The listing builds one solid part. Answer for the finished solid, in the listing's coordinates (mm). Face numbers are marked on the shaded views. A direction names the side the tool comes from. Coordinates: 2 decimals unless noted, no trailing zeros. Order: outer loops, then holes, each group sorted by start corner. A loop starts at its lowest first (then second) coordinate and runs counter-clockwise, first axis right, second up. Notation, with made-up numbers: (-27, 68.25) -> (27, 68.25) arc R24 ccw to (27, 100.25) -> close; hole circle Ø9 at (-5, 8.25). An arc over 180 degrees is marked (long way). One line per question, with ' | ' between items.
Autodesk Inventor part; units mm, degrees
ref_plane "YZ Plane" through (0, 0, 0) normal (1, 0, 0) x (0, 1, 0)
ref_plane "XZ Plane" through (0, 0, 0) normal (0, 1, 0) x (-1, 0, 0)
ref_plane "XY Plane" through (0, 0, 0) normal (0, 0, 1) x (1, 0, 0)
sketch "Sketch1" plane through (0, 0, 0) normal (0, 1, 0) x (-1, 0, 0)
  line L0 (-6, 6) -> (6, 6)
  line L1 (6, 6) -> (6, -6)
  line L2 (6, -6) -> (-6, -6)
  line L3 (-6, -6) -> (-6, 6)
  line L4 (-6, 6) -> (6, -6) construction
  line L5 (6, 6) -> (-6, -6) construction
  line L6 (6, 6) -> (16, 6)
  line L7 (16, -6) -> (6, -6)
  line L8 (6, -6) -> (6, 6)
  line L9 (0, 6) -> (0, -6) construction
  line L10 (-6, 6) -> (-16, 6)
  line L11 (-16, 6) -> (-16, -6)
  line L12 (-16, -6) -> (-6, -6)
  line L13 (-6, -6) -> (-6, -16)
  line L14 (-6, -16) -> (6, -16)
  line L15 (6, -16) -> (6, -6)
  line L16 (6, 6) -> (6, 16)
  line L17 (6, 16) -> (-6, 16)
  line L18 (-6, 16) -> (-6, 6)
  line L19 (16, 6) -> (16, -6)
  line L20 (6, 6) -> (-6, -6) construction
  line L21 (-6, 6) -> (6, -6) construction
  line L22 (-6, -6) -> (6, 6) construction
  circle A0 centre (0, 0) radius 6
  dimension "d0" = 12
  dimension "d1" = 12
  dimension "d6" = 12
  dimension "d38" = 12
  dimension "d39" = 10
  dimension "d40" = 10
extrude "Extrusion9" add sketch "Sketch1" along normal blind 6 contours L18 L17 L16 L0 | L0 A0 L3 | L3 L12 L11 L10 | L0 L1 A0 | A0 L2 L3 | L6 L19 L7 L1 | L1 L2 A0 | L2 L15 L14 L13
fillet "Fillet4" radius 6 4 edges at (-6, 3, -6) (6, 3, -6) (-6, 3, 6) (6, 3, 6)
sketch "Sketch11" plane through (16, 0, 6) normal (1, 0, 0) x (0, 0, -1)
  line L0 (6, 0) -> (6, 6)
  line L1 (0, 6) -> (12, 6)
  circle A0 centre (9, 3) radius 1
  line L2 (12, 0) -> (12, 6)
  line L3 (0, 0) -> (12, 0)
  circle A1 centre (3, 3) radius 1
  dimension "d69" = 2
  dimension "d70" = 3
  dimension "d71" = 3
hole "Hole1" at (16, 3, 3) at (16, 3, -3) direction (-1, 0, 0) diameter 1.567 depth 6.3 tip angle 118 countersink diameter 2.5 countersink angle 90
sketch "Sketch14" plane through (6, 0, -16) normal (0, 0, -1) x (-1, 0, 0)
  line L0 (6, 0) -> (6, 6)
  line L1 (0, 6) -> (12, 6)
  circle A0 centre (9, 3) radius 1
  line L2 (12, 0) -> (12, 6)
  line L3 (0, 0) -> (12, 0)
  circle A1 centre (3, 3) radius 1
  dimension "d99" = 2
  dimension "d100" = 3
  dimension "d101" = 3
hole "Hole2" at (3, 3, -16) at (-3, 3, -16) direction (0, 0, 1) diameter 1.567 depth 6.3 tip angle 118 countersink diameter 2.5 countersink angle 90
properties part number "rapoukMiddleLeg0v3" material "EN AW-6060 T6"
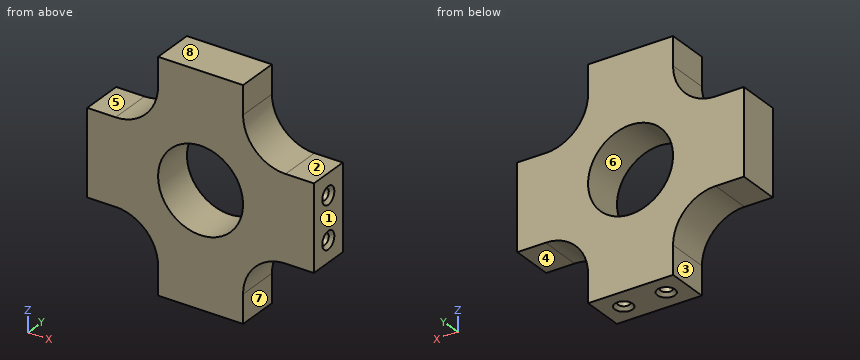
Item 1: Section C-C, the plane y = 0.9 is taken. Give the vertices of the cut face in (x, z).
Computed values:
outline: (-16, -6) -> (-12, -6) arc R6 cw to (-6, -12) -> (-6, -16) -> (6, -16) -> (6, -12) arc R6 cw to (12, -6) -> (16, -6) -> (16, 6) -> (12, 6) arc R6 cw to (6, 12) -> (6, 16) -> (-6, 16) -> (-6, 12) arc R6 cw to (-12, 6) -> (-16, 6) -> close; hole circle Ø12 at (0, 0)
Item 2: Section B-B, the plane z = -0.5 is taken. Give the vertices of the cut face in (x, y), plus the area to 3 significant figures.
Computed values:
outline: (-16, 0) -> (-5.98, 0) -> (-5.98, 6) -> (-16, 6) -> close; (5.98, 0) -> (16, 0) -> (16, 6) -> (5.98, 6) -> close | area: 120 mm^2
Item 3: Find the intervals of material crossed by L1, parallel to Z at x = 11.95, y = 3; L2, parallel to X at y = 4.3, z = 0; L3, parallel to Y at x = 3, z = -14.5, in increasing order.
Computed values:
L1: z = -6 to -3.78, -2.22 to 2.22, 3.78 to 6 | L2: x = -16 to -6, 6 to 16 | L3: y = 0 to 2.22, 3.78 to 6
Item 4: Determine the mould class of the marked faces 6, 7 and 8 for opening direction Z: pulls with the +Z half, pulls with the -Z half, needs draft (parallel to the pull), parting line crosses it, or undercut.
Computed values:
face 6: undercut | face 7: needs draft | face 8: pulls with the +Z half
Item 5: Section A-A, the plane x = 0 is taken. Give the vertices of the cut face in (y, z).
Computed values:
outline: (0, -16) -> (6, -16) -> (6, -6) -> (0, -6) -> close; (0, 6) -> (6, 6) -> (6, 16) -> (0, 16) -> close
Item 6: Section D-D, the plane x = -7.5 is taken. Give the vertices of the cut face in (y, z), plus the area to 3 significant figures.
Computed values:
outline: (0, -8.03) -> (6, -8.03) -> (6, 8.03) -> (0, 8.03) -> close | area: 96.4 mm^2
Item 7: For the marked faces 1, 2, 3, 4 and 5, determine the directions among +Z, -Z, +X, -X, +Y, -Y from which every point of the face is accessible in a straight line to the end or side of a thin tool.
Computed values:
face 1: +Z, -Z, +X, +Y, -Y | face 2: +Z, +X, +Y, -Y | face 3: -Z, -X, +Y, -Y | face 4: -Z, +X, +Y, -Y | face 5: +Z, -X, +Y, -Y
Item 8: Each of these flat-tipped pins is pushed along its axis until it touches: pin 1 Ø1.2 at (x, y) = (14, 2) entering from -Z; pin 2 Ø2 at (y, z) = (1.5, -15) entering from -X; pin 3 Ø1 at (x, y) = (11, 4) entering from +Z. Where does it stop, or does it pass through?
Computed values:
pin 1: stops at z = -6 | pin 2: stops at x = -6 | pin 3: stops at z = 6.19
